The listing builds one solid part. Answer for the finished solid, in the listing's coordinates (mm). Coordinates: 2 decimals unless noted, no trailing zeros. Order: outer loops, then holes, each group sorted by start corner. A loop starts at its lowest first (then second) coordinate and runs counter-clockwise, first axis right, second up.
from build123d import *

# Parameters (mm, degrees)
SKETCH1_W           = 70
SKETCH1_H           = 30
SKETCH1_R           = 12
SKETCH1_R_2         = 3.5
SKETCH1_W_2         = 15.5
SKETCH1_H_2         = 20.5
BOSS_EXTRUDE1_DEPTH = 2
FILLET1_R           = 0.5


with BuildPart() as part:
    # Sketch1 → Boss-Extrude1 (new body)
    with BuildSketch(Plane(origin=(0, 0, 0), x_dir=(1, 0, 0), z_dir=(0, 1, 0))):
        Rectangle(SKETCH1_W, SKETCH1_H)
        with Locations(Location((0, 0, 0), (0, 0, 270))):
            Circle(SKETCH1_R, mode=Mode.SUBTRACT)
        with Locations(Location((-20, 0, 0), (0, 0, 270))):
            Circle(SKETCH1_R_2, mode=Mode.SUBTRACT)
        with Locations((22, 0)):
            Rectangle(SKETCH1_W_2, SKETCH1_H_2, mode=Mode.SUBTRACT)
    extrude(amount=BOSS_EXTRUDE1_DEPTH)

    # Fillet1
    fillet1_edges = [part.edges().sort_by_distance(p)[0] for p in [
        (0, 0, -12),
        (0, 2, -12),
        (35, 2, 0),
        (-20, 0, -3.5),
        (-20, 2, -3.5),
        (0, 2, -15),
        (14.25, 0, 0),
        (22, 0, 10.25),
        (29.75, 0, 0),
        (22, 0, -10.25),
        (14.25, 2, 0),
        (22, 2, 10.25),
        (29.75, 2, 0),
        (22, 2, -10.25),
        (-35, 2, 0),
        (0, 0, -15),
        (35, 0, 0),
        (0, 0, 15),
        (-35, 0, 0),
        (0, 2, 15),
    ]]
    fillet(fillet1_edges, radius=FILLET1_R)


solid = part.part
1) Section C-C (x = -20) is taken. Give the vertices of the cut face in (y, z).
2) Section B-B (z = 0) is taken. Give the number of separate pieces and of enclosed holes in the cut face, then the cut area to 3 significant figures.
3) Section A-A (x = 19.5) is taken. Give the vertices of the cut face in (y, z).
4) Consider L1, parallel to X at y = 1.25, z = 0; L2, parallel to X at y = 0.15, z = 2.75; L3, parallel to X at y = 0.45, z = 7.75. Determine where each line is inside the solid, lowest interval first.
5) Determine the mould class of faces 1 (the face through (-16.53, 0.99, -0.46)), 2 (the face through (-15.8, 0, -0.2)) for opening direction Z: released by +Z, released by -Z, zero draft, split by the parting line, or undercut.
Filled sheet:
1. outline: (0, -14.5) arc R0.5 ccw to (0.5, -15) - (1.5, -15) arc R0.5 ccw to (2, -14.5) - (2, -4) arc R0.5 ccw to (1.5, -3.5) - (0.5, -3.5) arc R0.5 ccw to (0, -4) - close; (0, 4) arc R0.5 ccw to (0.5, 3.5) - (1.5, 3.5) arc R0.5 ccw to (2, 4) - (2, 14.5) arc R0.5 ccw to (1.5, 15) - (0.5, 15) arc R0.5 ccw to (0, 14.5) - close
2. separate pieces: 4
2. enclosed holes: 0
2. area: 46.1 mm2
3. outline: (0, -14.5) arc R0.5 ccw to (0.5, -15) - (1.5, -15) arc R0.5 ccw to (2, -14.5) - (2, -10.75) arc R0.5 ccw to (1.5, -10.25) - (0.5, -10.25) arc R0.5 ccw to (0, -10.75) - close; (0, 10.75) arc R0.5 ccw to (0.5, 10.25) - (1.5, 10.25) arc R0.5 ccw to (2, 10.75) - (2, 14.5) arc R0.5 ccw to (1.5, 15) - (0.5, 15) arc R0.5 ccw to (0, 14.5) - close
4. L1: x = -35 to -23.5, -16.5 to -12, 12 to 14.25, 29.75 to 35
4. L2: x = -34.86 to -22.39, -17.61 to -11.83, 11.83 to 14.11, 29.89 to 34.86
4. L3: x = -35 to -9.17, 9.17 to 14.25, 29.75 to 35
5. face 1: undercut
5. face 2: zero draft
